```python
from build123d import *

# Parameters (mm, degrees)
BOSS_EXTRUDE1_DEPTH = 6.35
CUT_EXTRUDE1_DEPTH  = 158.804246512
FILLET1_R           = 25.4


with BuildPart() as part:
    # Sketch1 → Boss-Extrude1 (new body)
    with BuildSketch(Plane(origin=(0, 0, 0), x_dir=(1, 0, 0), z_dir=(0, 1, 0))):
        with BuildLine():
            Line((7.9375, 111.6203), (7.9375, -4.582717762))
            Line((7.9375, -4.582717762), (-90.893507667, -61.642826643))
            ThreePointArc((-90.893507667, -61.642826643), (-101.73633431, -58.7375), (-98.831007667, -47.894673357))
            Line((-98.831007667, -47.894673357), (-7.9375, 4.582717762))
            Line((-7.9375, 4.582717762), (-7.9375, 111.6203))
            ThreePointArc((-7.9375, 111.6203), (0, 119.5578), (7.9375, 111.6203))
        make_face()
    extrude(amount=BOSS_EXTRUDE1_DEPTH)

    # Sketch2 → Cut-Extrude1 (cut, through all)
    with BuildSketch(Plane(origin=(0, 6.35, 0), x_dir=(1, 0, 0), z_dir=(0, 1, 0))):
        with BuildLine():
            Line((-90.893507667, -61.642826643), (-84.931832215, -58.200851716))
            ThreePointArc((-84.931832215, -58.200851716), (-90.389422779, -51.035617044), (-98.831007667, -47.894673357))
            ThreePointArc((-98.831007667, -47.894673357), (-101.73633431, -58.7375), (-90.893507667, -61.642826643))
        make_face()
    extrude(amount=-CUT_EXTRUDE1_DEPTH, mode=Mode.SUBTRACT)

    # Fillet1
    fillet1_edges = [part.edges().sort_by_distance(p)[0] for p in [
        (7.9375, 3.175, 4.582717762),
        (-7.9375, 3.175, -4.582717762),
    ]]
    fillet(fillet1_edges, radius=FILLET1_R)


solid = part.part
```
Geometry: final body of the model. Coordinates: model frame, mm. A direction names the side the tool comes from. Round coordinates to 2 decimals unless told otherwise and drop trailing zeros. Write each loop counter-clockwise with the first axis right and the second up, starting at its lowest first coordinate (ties: lowest second). Pieces come first, ordered by that corner, then holes. Notation, with made-up numbers: (77.5, -23.5) -> (117.5, -23.5) arc R17 cw to (117.5, -2.5) -> close; hole circle Ø3 at (14, 56). An arc over 180 degrees is marked (long way). Use CSV: the item, a comma, the result in double quotes. Start each with the question number.
Q1. First-contact query: pin 1 Ø3 at (y, z) = (4.5, -43.5) entering from -X; pin 2 Ø1 at (x, y) = (-85, 3) entering from -Z. Flat tips, straight axial feed; report the tip coordinate or a pass-through.
Q2. Line query: L1, parallel to X at y = 5.5, z = -22; L2, parallel to Z at x = -54.5, y = 3; L3, parallel to Z at x = -4, y = 4.5. Output: solid intervals per line, ascending.
Q3. Reachability of faces 4 (the face through (-90.3, 3.2, 51.1)), 5 (the face through (-7.938, 3, -65)) from +Z, -Z, +X, -X, +Y, -Y: full face, straight path, thin tool, end or side. Return the list, or none.
Q4. Section B-B (z = -93). Return loops of the section in (x, y).
Q5. Pull-direction query (X, two-part tool) for faces 1 (the face through (-44.286, 3.131, 34.734)), 2 (the face through (-6, 0, -18)), 3 (the face through (-60.282, 3.131, 25.638)); classes: pulls with the +X half, pulls with the -X half, needs draft (parallel to the pull), parting line crosses it, or undercut.
Q6. Section A-A (y = 4). Return loops of the section in (x, z) (1 decimal), plus the area to 3 significant figures.
Q7. Section C-C (x = 1). Return loops of the section in (y, z), plus the area to 3 significant figures.
Result sheet:
1,pin 1,"x = -7.94"
1,pin 2,"z = 39.62"
2,L1,"-7.94 to 7.94"
2,L2,"22.3 to 40.63"
2,L3,"-118.48 to 11.46"
3,face 4,"+Z, -X, +Y, -Y"
3,face 5,"-Z, -X, +Y, -Y"
4,outline,"(-7.94, 0) -> (7.94, 0) -> (7.94, 6.35) -> (-7.94, 6.35) -> close"
5,face 1,"pulls with the +X half"
5,face 2,"needs draft"
5,face 3,"pulls with the -X half"
6,outline,"(-98.8, 47.9) -> (-20.6, 2.7) arc R25.4 cw to (-7.9, -19.2) -> (-7.9, -111.6) arc R7.9 ccw to (7.9, -111.6) -> (7.9, -10.1) arc R25.4 ccw to (-4.8, 11.9) -> (-84.9, 58.2) arc R16.2 cw to start"
6,area,"3,530 mm²"
7,outline,"(0, -119.49) -> (6.35, -119.49) -> (6.35, 7.36) -> (0, 7.36) -> close"
7,area,"806 mm²"
